Geometry check sheet. Reference: the model listing, model coordinates, mm. A direction names the side the tool comes from. Round coordinates to 2 decimals unless told otherwise and drop trailing zeros. Write each loop counter-clockwise with the first axis right and the second up, starting at its lowest first coordinate (ties: lowest second). Pieces come first, ordered by that corner, then holes. Notation, with made-up numbers: (22, -7) - (65, -7) arc R36 ccw to (65, 30) - close; hole circle Ø5 at (-38, -37). An arc over 180 degrees is marked (long way). Return JSON: item names as keys, results as strings.
```python
from build123d import *

# Parameters (mm, degrees)
SKETCH1_W           = 220
SKETCH1_H           = 250
BOSS_EXTRUDE1_DEPTH = 5
SKETCH2_W           = 220
SKETCH2_H           = 250
SKETCH2_W_2         = 210
SKETCH2_H_2         = 73.333333333
SKETCH2_H_3         = 73.333333334
BOSS_EXTRUDE2_DEPTH = 140
SKETCH3_W           = 5
SKETCH3_H           = 5
CUT_EXTRUDE1_DEPTH  = 5
BOSS_EXTRUDE3_START = -5
BOSS_EXTRUDE3_DEPTH = 5


with BuildPart() as part:
    # Sketch1 → Boss-Extrude1 (new body)
    with BuildSketch(Plane(origin=(0, 0, 0), x_dir=(1, 0, 0), z_dir=(0, 1, 0))):
        Rectangle(SKETCH1_W, SKETCH1_H)
    extrude(amount=BOSS_EXTRUDE1_DEPTH)

    # Sketch2 → Boss-Extrude2 (add)
    with BuildSketch(Plane(origin=(0, 5, 0), x_dir=(1, 0, 0), z_dir=(0, 1, 0))):
        Rectangle(SKETCH2_W, SKETCH2_H)
        with Locations((0, 83.333333334)):
            Rectangle(SKETCH2_W_2, SKETCH2_H_2, mode=Mode.SUBTRACT)
        with Locations((0, -83.333333334)):
            Rectangle(SKETCH2_W_2, SKETCH2_H_2, mode=Mode.SUBTRACT)
        Rectangle(SKETCH2_W_2, SKETCH2_H_3, mode=Mode.SUBTRACT)
    extrude(amount=BOSS_EXTRUDE2_DEPTH)

    # Sketch3 → Cut-Extrude1 (cut)
    with BuildSketch(Plane.XY.offset(125)):
        Polygon((-105, 145), (-105, 77.5), (-105, 72.5), (-105, 5), (105, 5), (105, 72.5), (105, 77.5), (105, 145), align=None)
        with Locations((107.5, 75)):
            Rectangle(SKETCH3_W, SKETCH3_H)
        with Locations((-107.5, 75)):
            Rectangle(SKETCH3_W, SKETCH3_H)
    extrude(amount=-CUT_EXTRUDE1_DEPTH, mode=Mode.SUBTRACT)

    # Sketch4 → Boss-Extrude3 (add)
    with BuildSketch(Plane.XY.offset(-120).offset(BOSS_EXTRUDE3_START)):
        Polygon((105, 145), (-105, 145), (-105, 77.5), (-110, 77.5), (-110, 72.5), (-105, 72.5), (-105, 5), (105, 5), (105, 72.5), (110, 72.5), (110, 77.5), (105, 77.5), align=None)
    extrude(amount=-BOSS_EXTRUDE3_DEPTH)


solid = part.part
```
(1) Section check A-A, the plane y = 20. Enter the section's corners in (x, z).
Response values:
{"outline": "(-110, -125) - (-105, -125) - (-105, -130) - (105, -130) - (105, -125) - (110, -125) - (110, 125) - (105, 125) - (105, 46.67) - (-105, 46.67) - (-105, 125) - (-110, 125) - close; hole (-105, -120) - (105, -120) - (105, -46.67) - (-105, -46.67) - close; hole (-105, -36.67) - (105, -36.67) - (105, 36.67) - (-105, 36.67) - close"}
(2) Section check C-C, the plane x = -1. Enter the section's corners in (y, z).
Response values:
{"outline": "(0, -125) - (5, -125) - (5, -130) - (145, -130) - (145, -120) - (5, -120) - (5, -46.67) - (145, -46.67) - (145, -36.67) - (5, -36.67) - (5, 36.67) - (145, 36.67) - (145, 46.67) - (5, 46.67) - (5, 125) - (0, 125) - close"}
(3) Release check for a two-part mould opening along Z. For faces 4 (the face through (-2, 76, -130)), 5 (the face through (-9, 4, 125)), 6 (the face through (-1, 145, -41)), 7 (the face through (-1, 5, -1)) record: pulls with the +Z half, pulls with the -Z half, needs draft (parallel to the pull), parting line crosses it, or undercut.
Response values:
{"face 4": "pulls with the -Z half", "face 5": "pulls with the +Z half", "face 6": "needs draft", "face 7": "undercut"}
(4) Section check B-B, the plane z = -21.5. Enter the section's corners in (x, y), plus the area to 3 significant figures.
Response values:
{"outline": "(-110, 0) - (110, 0) - (110, 145) - (105, 145) - (105, 5) - (-105, 5) - (-105, 145) - (-110, 145) - close", "area": "2,500 mm^2"}
(5) Material ranges on line 1 along Z through (x, y) = (51, 36.5); line 2 along X through (y, z) = (10.5, 55); line 3 along Y through (x, z) = (81, -28), recorded low to high. Write a range as [from, to].
Response values:
{"line 1": "z = [-130, -120], [-46.67, -36.67], [36.67, 46.67]", "line 2": "x = [-110, -105], [105, 110]", "line 3": "y = [0, 5]"}
(6) Gauge pin test, flat ends, axial feed: pin 1 (4 mm diameter, centred on x = 21.5, y = 98, fed in from +Z); pin 2 (1.5 mm diameter, centred on x = -79, z = 98.5, fed in from +Y); pin 3 (2.5 mm diameter, centred on y = 103.5, z = -127.5, fed in from -X). Record the tip position at first contact, or that the pin passes through.
Response values:
{"pin 1": "stops at z = 46.67", "pin 2": "stops at y = 5", "pin 3": "stops at x = -105"}
(7) Access from +Z, -Z, +X, -X, +Y, -Y to the whole of each face (thin tool, end or side, straight path). Record for faces 1 (the face through (105, 74, 1)), 2 (the face through (-110, 71, -1)), 3 (the face through (-1, 74, 46.667)).
Response values:
{"face 1": "+Y", "face 2": "+Z, -Z, -X, +Y, -Y", "face 3": "+Z, +Y"}
